Build history of the part. All positions in model axes, mm. Face numbers are marked on the shaded views. A direction names the side the tool comes from. Give positions to 0.01 mm unless a question says otherwise; leave off trailing zeros. Order: outer loops, then holes, each group sorted by start corner. A loop starts at its lowest first (then second) coordinate and runs counter-clockwise, first axis right, second up. Notation, with made-up numbers: (-38, 26.25) - (-1, 26.25) arc R17 ccw to (-1, 33.25) - close; hole circle Ø6 at (49.25, 53). An arc over 180 degrees is marked (long way). Answer in a Markdown table with one row per item.
```python
from build123d import *

# Parameters (mm, degrees)
SKETCH_1_R      = 10
EXTRUDE_3_DEPTH = 5
SKETCH_3_R      = 5
EXTRUDE_4_DEPTH = 5
SKETCH_4_R      = 5
EXTRUDE_5_DEPTH = 5


with BuildPart() as part:
    # 草图1 → 凸台-拉伸3 (new body)
    with BuildSketch(Plane.XY):
        Circle(SKETCH_1_R)
        with BuildLine():
            Line((51.049932735, 4.46052642), (8.950067265, 4.46052642))
            ThreePointArc((8.950067265, 4.46052642), (9.733978443, 2.291214454), (10, 0))
            ThreePointArc((10, 0), (9.733978443, -2.291214454), (8.950067265, -4.46052642))
            Line((8.950067265, -4.46052642), (51.049932735, -4.46052642))
            ThreePointArc((51.049932735, -4.46052642), (50, 0), (51.049932735, 4.46052642))
        make_face()
        with Locations((60, 0)):
            Circle(SKETCH_1_R)
    extrude(amount=EXTRUDE_3_DEPTH)

    # 草图3 → 凸台-拉伸4 (add)
    with BuildSketch(Plane.XY.offset(5)):
        with Locations((60, 0)):
            Circle(SKETCH_3_R)
    extrude(amount=EXTRUDE_4_DEPTH)

    # 草图4 → 凸台-拉伸5 (add)
    with BuildSketch(Plane.XY.offset(5)):
        Circle(SKETCH_4_R)
    extrude(amount=EXTRUDE_5_DEPTH)


solid = part.part
```
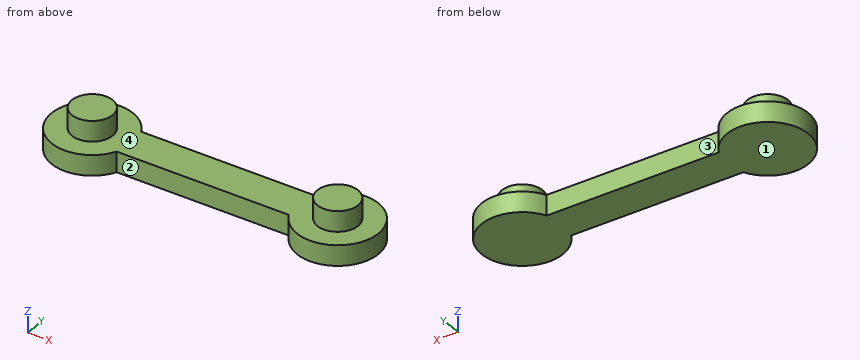
1. Cut at D-D on z = 3.75. Write the cut outline in (x, y), and give its area (3 significant figures).
Check result:
| item | result |
|---|---|
| outline | (8.95, -4.46) - (51.05, -4.46) arc R10 ccw (long way) to (51.05, 4.46) - (8.95, 4.46) arc R10 ccw (long way) to start |
| area | 991 mm² |
2. Cut at B-B on y = 0. Write the cut outline in (x, z), and give its area (3 significant figures).
Check result:
| item | result |
|---|---|
| outline | (-10, 0) - (70, 0) - (70, 5) - (65, 5) - (65, 10) - (55, 10) - (55, 5) - (5, 5) - (5, 10) - (-5, 10) - (-5, 5) - (-10, 5) - close |
| area | 500 mm² |
3. Cut at C-C on z = 9.25. Write the cut outline in (x, y), and give its area (3 significant figures).
Check result:
| item | result |
|---|---|
| outline | circle Ø10 at (0, 0); circle Ø10 at (60, 0) |
| area | 157 mm² |
4. Probe line 1 (Y direction, x = 15, z = 2); line 2 (Z direction, x = 31, y = 3.5); line 3 (X direction, y = 7, z = 1.5). List the from-to ranges inside material, lowest first.
Check result:
| item | result |
|---|---|
| line 1 | y = -4.46 to 4.46 |
| line 2 | z = 0 to 5 |
| line 3 | x = -7.14 to 7.14, 52.86 to 67.14 |
5. Cut at A-A on x = 60. Write the cut outline in (y, z), and give its area (3 significant figures).
Check result:
| item | result |
|---|---|
| outline | (-10, 0) - (10, 0) - (10, 5) - (5, 5) - (5, 10) - (-5, 10) - (-5, 5) - (-10, 5) - close |
| area | 150 mm² |
6. Drop flat-ended pins along their axis: P1, Ø5.5, axis at x = 33, z = 2, coming from the +Y side; P2, Ø6, axis at x = 5, z = 5, coming from the -Y side; P3, Ø5.5, axis at x = 25, z = 2.5, coming from the -Y side. Give the stop position or say it passes through.
Check result:
| item | result |
|---|---|
| P1 | stops at y = 4.46 |
| P2 | stops at y = -9.8 |
| P3 | stops at y = -4.46 |
7. Which spindle directions (+Z, -Z, +X, -X, +Y, -Y) get a long thin tool onto all of the face, cutting with end or side? Do the marked faces 1, 2, 3 and 4. Say none if no direction does.
Check result:
| item | result |
|---|---|
| face 1 | -Z, +X, -X, +Y, -Y |
| face 2 | +Z, -Z, -Y |
| face 3 | +Z, -Z, +Y |
| face 4 | +Z |
